The model under review builds one solid part; all positions refer to its coordinate system, in mm. A direction names the side the tool comes from. Round coordinates to 2 decimals unless told otherwise and drop trailing zeros. Order: outer loops, then holes, each group sorted by start corner. A loop starts at its lowest first (then second) coordinate and runs counter-clockwise, first axis right, second up. Notation, with made-up numbers: (23, -3) -> (46, -3) arc R24 ccw to (46, 17) -> close; hole circle Ø4 at (1, 61). An arc over 180 degrees is marked (long way). Use a Markdown table: item, result. Add a question column.
```python
from build123d import *

# Parameters (mm, degrees)
CHAFL_N2_SIZE = 1


with BuildPart() as part:
    # Croquis1 → Revolución1 (revolve)
    with BuildSketch(Plane.XY, mode=Mode.PRIVATE) as revoluci_n1_sk:
        Polygon((12, -11.11234319), (12, 87.88765681), (9.75, 87.88765681), (0, 87.88765681), (0, -15.61234319), (7.5, -15.61234319), align=None)
    revolve(revoluci_n1_sk.sketch.rotate(Axis((0, 0, 0), (0, 1, 0)), 90), axis=Axis((0, 0, 0), (0, 1, 0)))

    # Chaflán2
    chafl_n2_edges = [part.edges().sort_by_distance(p)[0] for p in [
        (0, 87.88765681, 12),
    ]]
    chamfer(chafl_n2_edges, length=CHAFL_N2_SIZE)

    # Croquis2 → Revolución2 (revolve)
    with BuildSketch(Plane.XY, mode=Mode.PRIVATE) as revoluci_n2_sk:
        Polygon((0, 87.88765681), (9.75, 87.88765681), (9.75, 106.88765681), (6, 135.88765681), (4, 135.88765681), (4, 185.88765681), (0, 185.88765681), (0, 135.88765681), align=None)
    revolve(revoluci_n2_sk.sketch.rotate(Axis((0, 135.88765681, 0), (0, -1, 0)), 90), axis=Axis((0, 135.88765681, 0), (0, -1, 0)))


solid = part.part
```
Q1. For faces 1 (the face through (-3.604, 38.574, -11.446)), 2 (the face through (10, 87.888, 1)), list the 3-axis set-ups (+Z, -Z, +X, -X, +Y, -Y) from which the entire face can be reached by the end or side of a thin tool; tool diameter is ignored.
Q2. To check wall thickness, follow line 1 along Z through (x, y) = (0.25, 105); line 2 along Y through (x, z) = (-2.75, -4.5). State the ranges of each line that lie inside material, in increasing order.
Q3. For pin 1 (12 mm diameter, centred on x = -8, y = 12.5, fed in from +Z); pin 2 (10 mm diameter, centred on y = 131, z = -6.5, fed in from -X); pin 3 (3 mm diameter, centred on x = -1, y = 136.5, fed in from +Z), all flat-tipped, find the tip position at first contact; note any pin that passes through.
Q4. Add section C-C, the plane y = 165.5. Give the boundary of the cut face in (x, z), then the cut area to 3 significant figures.
Q5. Add section B-B, the plane x = 0. Give the boundary of the cut face in (y, z).
Q6. Add section D-D, the plane y = 93.5. Give the boundary of the cut face in (x, z), then the cut area to 3 significant figures.
Q7. Add section A-A, the plane z = 0. Give the boundary of the cut face in (x, y).
Return value:
| question | item | result |
|---|---|---|
| 1 | face 1 | +Y, -Y |
| 1 | face 2 | +Y |
| 2 | line 1 | -9.75 to 9.75 |
| 2 | line 2 | -15.61 to 135.89 |
| 3 | pin 1 | z = 11.83 |
| 3 | pin 2 | x = -6.62 |
| 3 | pin 3 | z = 6.09 |
| 4 | outline | circle Ø8 at (0, 0) |
| 4 | area | 50.3 mm² |
| 5 | outline | (-15.61, -7.5) -> (-11.11, -12) -> (86.89, -12) -> (87.89, -11) -> (87.89, -9.75) -> (106.89, -9.75) -> (135.89, -6) -> (135.89, -4) -> (185.89, -4) -> (185.89, 4) -> (135.89, 4) -> (135.89, 6) -> (106.89, 9.75) -> (87.89, 9.75) -> (87.89, 11) -> (86.89, 12) -> (-11.11, 12) -> (-15.61, 7.5) -> close |
| 6 | outline | circle Ø19.5 at (0, 0) |
| 6 | area | 299 mm² |
| 7 | outline | (-12, -11.11) -> (-7.5, -15.61) -> (7.5, -15.61) -> (12, -11.11) -> (12, 86.89) -> (11, 87.89) -> (9.75, 87.89) -> (9.75, 106.89) -> (6, 135.89) -> (4, 135.89) -> (4, 185.89) -> (-4, 185.89) -> (-4, 135.89) -> (-6, 135.89) -> (-9.75, 106.89) -> (-9.75, 87.89) -> (-11, 87.89) -> (-12, 86.89) -> close |
